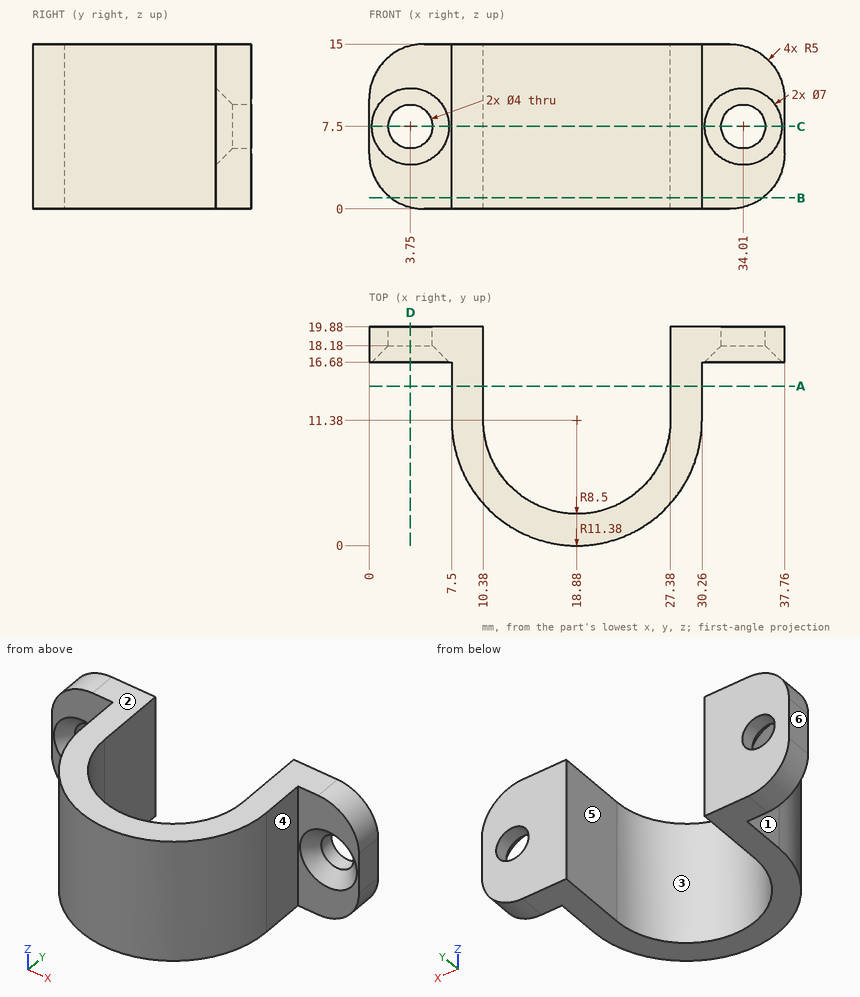
Input: dimensioned drawing with shaded views. Units: mm. Origin: part minimum x, y, z. A direction names the side the tool comes from. Round coordinates to 2 decimals unless told otherwise and drop trailing zeros. Loops run counter-clockwise (first coordinate to the right, second up) from the corner with the lowest first, then second, coordinate; pieces in that order, holes last.
1) Section query B-B on z = 1. Return the cut outline in (x, y).
Ans:
outline: (2, 16.68) - (7.5, 16.68) - (7.5, 11.38) arc R11.38 ccw to (30.26, 11.38) - (30.26, 16.68) - (35.76, 16.68) - (35.76, 19.88) - (27.38, 19.88) - (27.38, 11.38) arc R8.5 cw to (10.38, 11.38) - (10.38, 19.88) - (2, 19.88) - close
2) Section query D-D on x = 3.75. Return the cut outline in (y, z).
Ans:
outline: (16.68, 0.16) - (19.88, 0.16) - (19.88, 5.5) - (18.18, 5.5) - (16.68, 4) - close; (16.68, 11) - (18.18, 9.5) - (19.88, 9.5) - (19.88, 14.84) - (16.68, 14.84) - close
3) Section query C-C on z = 7.5. Return the cut outline in (x, y).
Ans:
outline: (0, 16.68) - (0.25, 16.68) - (1.75, 18.18) - (1.75, 19.88) - (0, 19.88) - close; (5.75, 18.18) - (7.25, 16.68) - (7.5, 16.68) - (7.5, 11.38) arc R11.38 ccw to (30.26, 11.38) - (30.26, 16.68) - (30.51, 16.68) - (32.01, 18.18) - (32.01, 19.88) - (27.38, 19.88) - (27.38, 11.38) arc R8.5 cw to (10.38, 11.38) - (10.38, 19.88) - (5.75, 19.88) - close; (36.01, 18.18) - (37.51, 16.68) - (37.76, 16.68) - (37.76, 19.88) - (36.01, 19.88) - close
4) Pin query (flat end, axial travel): pin 1 (2 mm diameter, centred on x = 30.5, y = 4, fed in from +Z); pin 2 (6 mm diameter, centred on y = 13.5, z = 10.5, fed in from -X); pin 3 (6 mm diameter, centred on x = 2.5, z = 10, fed in from -Y); pin 4 (1.6 mm diameter, centred on y = 14, z = 6, fed in from +X). Return the tip coordinate at first contact, or that it passes through.
Ans:
pin 1: passes through
pin 2: stops at x = 7.5
pin 3: stops at y = 16.68
pin 4: stops at x = 30.26
5) Set-up query: the marked faces 4, 5 and 6. Return all of +Z, -Z, +X, -X, +Y, -Y with unobstructed straight access to the full face (end or side cutting, diameter ignored); none if empty.
Ans:
face 4: +Z, -Z, +X, -Y
face 5: +Z, -Z, +Y
face 6: +Z, -Z, -X, +Y, -Y
6) Material intervals for line 1 (X direction, y = 19.35, z = 7.5); line 2 (X direction, y = 13.25, z = 1); line 3 (X direction, y = 17.5, z = 4.5), sorted ascending.
Ans:
line 1: x = 0 to 1.75, 5.75 to 10.38, 27.38 to 32.01, 36.01 to 37.76
line 2: x = 7.5 to 10.38, 27.38 to 30.26
line 3: x = 0.03 to 10.38, 27.38 to 37.73
7) Section query A-A on y = 14.5. Return the cut outline in (x, z).
Ans:
outline: (7.5, 0) - (10.38, 0) - (10.38, 15) - (7.5, 15) - close; (27.38, 0) - (30.26, 0) - (30.26, 15) - (27.38, 15) - close
8) Pull-direction query (X, two-part tool) for the marked faces 1, 2 and 3; classes: released by +X, released by -X, zero draft, split by the parting line, or undercut.
Ans:
face 1: released by -X
face 2: zero draft
face 3: undercut
